from build123d import *

# Parameters (mm, degrees)
SKETCH1_W                                       = 140
SKETCH1_H                                       = 180
BOSS_EXTRUDE1_DEPTH                             = 12.7
CSK_FOR_M4_FLAT_HEAD_MACHINE_SCREW1_D           = 4.5
CSK_FOR_M4_FLAT_HEAD_MACHINE_SCREW1_CSINK_D     = 9.4
CSK_FOR_M4_FLAT_HEAD_MACHINE_SCREW1_CSINK_ANGLE = 90


with BuildPart() as part:
    # Sketch1 → Boss-Extrude1 (new body)
    with BuildSketch(Plane(origin=(0, 0, 0), x_dir=(1, 0, 0), z_dir=(0, 1, 0))):
        Rectangle(SKETCH1_W, SKETCH1_H)
    extrude(amount=BOSS_EXTRUDE1_DEPTH)

    # CSK for M4 Flat Head Machine Screw1 (through all)
    with Locations(Plane(origin=(0, 12.7, 0), x_dir=(1, 0, 0), z_dir=(0, 1, 0))):
        with Locations((0, -52.5), (30, -52.5), (31.487677762, -77.5), (0, -77.5), (0, 77.5), (30, 77.5), (31.487677762, 52.5), (0, 52.5)):
            CounterSinkHole(CSK_FOR_M4_FLAT_HEAD_MACHINE_SCREW1_D / 2, CSK_FOR_M4_FLAT_HEAD_MACHINE_SCREW1_CSINK_D / 2, counter_sink_angle=CSK_FOR_M4_FLAT_HEAD_MACHINE_SCREW1_CSINK_ANGLE)


solid = part.part
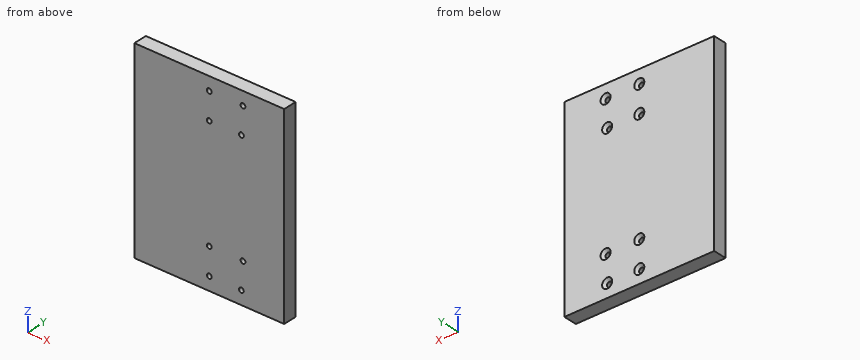
Verification items for the finished model (mm, model axes). Give positions to 0.01 mm unless a question says otherwise; leave off trailing zeros. Order: outer loops, then holes, each group sorted by start corner. A loop starts at its lowest first (then second) coordinate and runs counter-clockwise, first axis right, second up. Notation, with made-up numbers: (-10, 58) -> (12, 58) arc R23 ccw to (12, 75) -> close; hole circle Ø9 at (-10.5, 5). An arc over 180 degrees is marked (long way). Answer as CSV lines item,"result".
Q1. Depth check by flat-ended pin: pin 1 (7 mm diameter, centred on x = 31.49, z = 77.5, fed in from +Y); pin 2 (2.5 mm diameter, centred on x = 30, z = 52.5, fed in from +Y); pin 3 (5 mm diameter, centred on x = 31.49, z = -52.5, fed in from +Y). Enter the tip coordinate at first touch or a pass-through.
Solutions:
pin 1,"stops at y = 11.5"
pin 2,"passes through"
pin 3,"stops at y = 10.5"
Q2. Sectioned sample at B-B on z = -77.5. Record the cut outline in (x, y).
Solutions:
outline,"(-70, 0) -> (-2.25, 0) -> (-2.25, 10.25) -> (-4.7, 12.7) -> (-70, 12.7) -> close; (2.25, 0) -> (27.75, 0) -> (27.75, 10.25) -> (25.3, 12.7) -> (4.7, 12.7) -> (2.25, 10.25) -> close; (32.25, 0) -> (70, 0) -> (70, 12.7) -> (34.7, 12.7) -> (32.25, 10.25) -> close"
Q3. Scan lines: probe 1 along Z at (x, y) = (0, 3.5); probe 2 along X at (y, z) = (10.25, -75.5); probe 3 along X at (y, z) = (7, 77.5). Record each from-to range of solid material in increasing order.
Solutions:
probe 1,"z = -90 to -79.75, -75.25 to -54.75, -50.25 to 50.25, 54.75 to 75.25, 79.75 to 90"
probe 2,"x = -70 to -1.03, 1.03 to 28.97, 31.03 to 70"
probe 3,"x = -70 to -2.25, 2.25 to 29.24, 33.74 to 70"
Q4. Sectioned sample at A-A on x = 0. Record the cut outline in (y, z).
Solutions:
outline,"(0, -90) -> (12.7, -90) -> (12.7, -82.2) -> (10.25, -79.75) -> (0, -79.75) -> close; (0, -75.25) -> (10.25, -75.25) -> (12.7, -72.8) -> (12.7, -57.2) -> (10.25, -54.75) -> (0, -54.75) -> close; (0, -50.25) -> (10.25, -50.25) -> (12.7, -47.8) -> (12.7, 47.8) -> (10.25, 50.25) -> (0, 50.25) -> close; (0, 54.75) -> (10.25, 54.75) -> (12.7, 57.2) -> (12.7, 72.8) -> (10.25, 75.25) -> (0, 75.25) -> close; (0, 79.75) -> (10.25, 79.75) -> (12.7, 82.2) -> (12.7, 90) -> (0, 90) -> close"
